Part model, mm, in its own coordinate system. Coordinates: 2 decimals unless noted, no trailing zeros. Write each loop counter-clockwise with the first axis right and the second up, starting at its lowest first coordinate (ties: lowest second). Pieces come first, ordered by that corner, then holes. Notation, with made-up numbers: (37.5, 5.25) -> (46.5, 5.25) arc R22 cw to (46.5, 42.25) -> close; hole circle Ø1 at (-33.75, -19.5). An arc over 180 degrees is marked (long way). Write item = value, one per line.
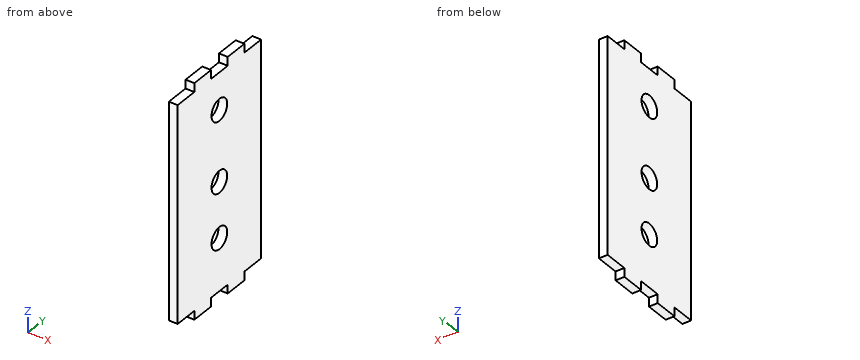
from build123d import *

# Parameters (mm, degrees)
CROQUIS1_W              = 160
CROQUIS1_H              = 80
SALIENTE_EXTRUIR1_DEPTH = 6
CROQUIS2_R              = 7.5
CORTAR_EXTRUIR1_DEPTH   = 6
CROQUIS3_W              = 6
CROQUIS3_H              = 16
CORTAR_EXTRUIR2_DEPTH   = 6


with BuildPart() as part:
    # Croquis1 → Saliente-Extruir1 (new body)
    with BuildSketch(Plane(origin=(0, 0, 0), x_dir=(0, 0, -1), z_dir=(1, 0, 0))):
        Rectangle(CROQUIS1_W, CROQUIS1_H)
    extrude(amount=SALIENTE_EXTRUIR1_DEPTH)

    # Croquis2 → Cortar-Extruir1 (cut)
    with BuildSketch(Plane(origin=(6, 0, 0), x_dir=(0, 0, -1), z_dir=(1, 0, 0))):
        with Locations((-48.61, 0)):
            Circle(CROQUIS2_R)
        Circle(CROQUIS2_R)
        with Locations((38.1, 0)):
            Circle(CROQUIS2_R)
    extrude(amount=-CORTAR_EXTRUIR1_DEPTH, mode=Mode.SUBTRACT)

    # Croquis3 → Cortar-Extruir2 (cut)
    with BuildSketch(Plane(origin=(6, 0, 0), x_dir=(0, 0, -1), z_dir=(1, 0, 0))):
        with Locations((-77, 32)):
            Rectangle(CROQUIS3_W, CROQUIS3_H)
        with Locations((-77, -32)):
            Rectangle(CROQUIS3_W, CROQUIS3_H)
        with Locations((77, -32)):
            Rectangle(CROQUIS3_W, CROQUIS3_H)
        with Locations((77, 32)):
            Rectangle(CROQUIS3_W, CROQUIS3_H)
        with Locations((77, 0)):
            Rectangle(CROQUIS3_W, CROQUIS3_H)
        with Locations((-77, 0)):
            Rectangle(CROQUIS3_W, CROQUIS3_H)
    extrude(amount=-CORTAR_EXTRUIR2_DEPTH, mode=Mode.SUBTRACT)


solid = part.part
Q1. Probe line 1 (Y direction, x = 2.25, z = 48.61); line 2 (Z direction, x = 3.4, y = 27); line 3 (Y direction, x = 4.3, z = 6). List the from-to ranges inside material, lowest first. Write a range as from..to.
Model answer:
line_1 = -40..-7.5, 7.5..40
line_2 = -74..74
line_3 = -40..-4.5, 4.5..40
Q2. Saw through at B-B on z = 0. Give the cut face in (x, y), and give its area (3 significant figures).
Model answer:
outline = (0, -40) -> (6, -40) -> (6, -7.5) -> (0, -7.5) -> close; (0, 7.5) -> (6, 7.5) -> (6, 40) -> (0, 40) -> close
area = 390 mm²
Q3. Saw through at C-C on x = 1.75. Give the cut face in (y, z), and give its area (3 significant figures).
Model answer:
outline = (-40, -74) -> (-24, -74) -> (-24, -80) -> (-8, -80) -> (-8, -74) -> (8, -74) -> (8, -80) -> (24, -80) -> (24, -74) -> (40, -74) -> (40, 74) -> (24, 74) -> (24, 80) -> (8, 80) -> (8, 74) -> (-8, 74) -> (-8, 80) -> (-24, 80) -> (-24, 74) -> (-40, 74) -> close; hole circle Ø15 at (0, -38.1); hole circle Ø15 at (0, 0); hole circle Ø15 at (0, 48.61)
area = 11,700 mm²
Q4. Pin check, flat tips, straight feed: pin 1 (3 mm diameter, centred on x = 2, z = 76.5, fed in from -Y); pin 2 (2 mm diameter, centred on x = 2, y = -1.5, fed in from -Z); pin 3 (1.8 mm diameter, centred on x = 2, z = -76.5, fed in from +Y). Stop position of each tip, or through.
Model answer:
pin_1 = -24
pin_2 = -74
pin_3 = 24
Q5. Saw through at A-A on y = 0. Give the cut face in (x, z), and give its area (3 significant figures).
Model answer:
outline = (0, -74) -> (6, -74) -> (6, -45.6) -> (0, -45.6) -> close; (0, -30.6) -> (6, -30.6) -> (6, -7.5) -> (0, -7.5) -> close; (0, 7.5) -> (6, 7.5) -> (6, 41.11) -> (0, 41.11) -> close; (0, 56.11) -> (6, 56.11) -> (6, 74) -> (0, 74) -> close
area = 618 mm²
Q6. Saw through at D-D on z = -35. Give the cut face in (x, y).
Model answer:
outline = (0, -40) -> (6, -40) -> (6, -6.83) -> (0, -6.83) -> close; (0, 6.83) -> (6, 6.83) -> (6, 40) -> (0, 40) -> close
